Read the model definition and answer for the solid it produces. Units are mm, in the model's axes. A direction names the side the tool comes from. Give positions to 0.01 mm unless a question says otherwise; leave off trailing zeros. Order: outer loops, then holes, each group sorted by start corner. A loop starts at its lowest first (then second) coordinate and runs counter-clockwise, first axis right, second up. Notation, with made-up numbers: M 39,-1.75 L 70,-1.75 A34 ccw 70,29.25 Z; hole C 19,83.5 d5. An arc over 180 degrees is marked long. Write item = value, one per line. Start each with the question number.
from build123d import *

# Parameters (mm, degrees)
SKETCH2_W           = 120
SKETCH2_H           = 105
SKETCH2_R           = 1.4
BOSS_EXTRUDE2_DEPTH = 5
CUT_EXTRUDE13_DEPTH = 90.336442732
FILLET6_R           = 5
FILLET5_R           = 10
CHAMFER4_SIZE       = 1
SKETCH11_R          = 2.15
CUT_EXTRUDE10_DEPTH = 90.336442732
SKETCH13_R          = 3.25
CUT_EXTRUDE12_DEPTH = 2.5
CUT_EXTRUDE14_DEPTH = 90.336442732
CHAMFER5_SIZE       = 3
CHAMFER5_SIZE_2     = 8.242432258


with BuildPart() as part:
    # Sketch2 → Boss-Extrude2 (new body)
    with BuildSketch(Plane(origin=(0, 0, 0), x_dir=(1, 0, 0), z_dir=(0, 1, 0))):
        with Locations((0, 13.5)):
            Rectangle(SKETCH2_W, SKETCH2_H)
        with Locations(Location((-28, -28, 0), (0, 0, 270))):
            Circle(SKETCH2_R, mode=Mode.SUBTRACT)
        with Locations(Location((28, -28, 0), (0, 0, 270))):
            Circle(SKETCH2_R, mode=Mode.SUBTRACT)
        with Locations(Location((20, 42, 0), (0, 0, 270))):
            Circle(SKETCH2_R, mode=Mode.SUBTRACT)
        with Locations(Location((-20, 42, 0), (0, 0, 270))):
            Circle(SKETCH2_R, mode=Mode.SUBTRACT)
    extrude(amount=BOSS_EXTRUDE2_DEPTH)

    # Sketch9 → Cut-Extrude13 (cut, through all)
    with BuildSketch(Plane(origin=(0, 5, 0), x_dir=(1, 0, 0), z_dir=(0, 1, 0))):
        Polygon((-26, 66), (-20, 60), (20, 60), (26, 66), align=None)
    extrude(amount=-CUT_EXTRUDE13_DEPTH, mode=Mode.SUBTRACT)

    # Fillet6
    fillet6_edges = [part.edges().sort_by_distance(p)[0] for p in [
        (-26, 2.5, -66),
        (26, 2.5, -66),
        (20, 2.5, -60),
        (-20, 2.5, -60),
    ]]
    fillet(fillet6_edges, radius=FILLET6_R)

    # Fillet5
    fillet5_edges = [part.edges().sort_by_distance(p)[0] for p in [
        (-60, 2.5, -66),
        (60, 2.5, -66),
        (60, 2.5, 39),
        (-60, 2.5, 39),
    ]]
    fillet(fillet5_edges, radius=FILLET5_R)

    # Chamfer4
    chamfer4_edges = [part.edges().sort_by_distance(p)[0] for p in [
        (23, 5, -63),
        (0, 5, -60),
        (-23, 5, -63),
        (-39.035533906, 5, -66),
        (-26.15765065, 5, -65.619397663),
        (26.15765065, 5, -65.619397663),
        (19.84234935, 5, -60.380602337),
        (-19.84234935, 5, -60.380602337),
        (-60, 5, -13.5),
        (39.035533906, 5, -66),
        (0, 5, 39),
        (60, 5, -13.5),
        (-57.071067812, 5, 36.071067812),
        (57.071067812, 5, 36.071067812),
        (57.071067812, 5, -63.071067812),
        (-57.071067812, 5, -63.071067812),
    ]]
    chamfer(chamfer4_edges, length=CHAMFER4_SIZE)

    # Sketch11 → Cut-Extrude10 (cut, through all)
    with BuildSketch(Plane(origin=(0, 5, 0), x_dir=(1, 0, 0), z_dir=(0, 1, 0))):
        with Locations(Location((-50, 56, 0), (0, 0, 270))):
            Circle(SKETCH11_R)
        with Locations(Location((50, 56, 0), (0, 0, 270))):
            Circle(SKETCH11_R)
        with Locations(Location((-50, -19, 0), (0, 0, 270))):
            Circle(SKETCH11_R)
        with Locations(Location((50, -19, 0), (0, 0, 270))):
            Circle(SKETCH11_R)
    extrude(amount=-CUT_EXTRUDE10_DEPTH, mode=Mode.SUBTRACT)

    # Sketch13 → Cut-Extrude12 (cut)
    with BuildSketch(Plane.XZ):
        with Locations(Location((-28, 28, 0), (0, 0, 270))):
            Circle(SKETCH13_R)
        with Locations(Location((28, 28, 0), (0, 0, 270))):
            Circle(SKETCH13_R)
        with Locations(Location((-20, -42, 0), (0, 0, 270))):
            Circle(SKETCH13_R)
        with Locations(Location((20, -42, 0), (0, 0, 270))):
            Circle(SKETCH13_R)
    extrude(amount=-CUT_EXTRUDE12_DEPTH, mode=Mode.SUBTRACT)

    # Sketch14 → Cut-Extrude14 (cut, through all)
    with BuildSketch(Plane(origin=(0, 5, 0), x_dir=(1, 0, 0), z_dir=(0, 1, 0))):
        with BuildLine():
            Line((-11, 38), (11, 38))
            ThreePointArc((11, 38), (18, 31), (11, 24))
            Line((11, 24), (-11, 24))
            ThreePointArc((-11, 24), (-18, 31), (-11, 38))
        make_face()
    extrude(amount=-CUT_EXTRUDE14_DEPTH, mode=Mode.SUBTRACT)

    # Chamfer5
    # the kernel refuses this chamfer: 8.242432258, 3 mm, written as the material it takes off along each edge
    with BuildSketch(Plane(origin=(11, 5, -24), x_dir=(0, 0.09904090225205062, 0.9950833631817486), z_dir=(-1, 0, 0)), Plane(origin=(-11, 5, -38), x_dir=(0, 0.09904090225205073, -0.9950833631817486), z_dir=(1, 0, 0))) as chamfer5_piece_1:
        Polygon((CHAMFER5_SIZE * 0.995083363182, -CHAMFER5_SIZE * 0.0990409022521), (-CHAMFER5_SIZE_2 * 0.0990409022564, -CHAMFER5_SIZE_2 * 0.995083363226), (0, 0), align=None)
    extrude(amount=22, mode=Mode.SUBTRACT)
    with BuildSketch(Plane(origin=(11, 5, -31), x_dir=(0, 0, -1), z_dir=(-1, 0, 0))) as chamfer5_piece_2:
        Polygon((7 + CHAMFER5_SIZE, 0), (7, CHAMFER5_SIZE_2), (7, 0), align=None)
    revolve(axis=Axis((11, 5, -31), (0, -1, 0)), revolution_arc=180, mode=Mode.SUBTRACT)
    with BuildSketch(Plane(origin=(-11, 5, -31), x_dir=(0, 0, 1), z_dir=(1, 0, 0))) as chamfer5_piece_3:
        Polygon((7 + CHAMFER5_SIZE, 0), (7, CHAMFER5_SIZE_2), (7, 0), align=None)
    revolve(axis=Axis((-11, 5, -31), (0, -1, 0)), revolution_arc=180, mode=Mode.SUBTRACT)


solid = part.part
1) Find section A-A on z = -31. Determine the outline of the cut face in (x, y).
2) Find section B-B on x = 9. Determine the outline of the cut face in (y, z), plus the area to 3 significant figures.
3) For a pull along X with two mould halves and no side action, classify faces 6 (the face through (-56.558, 4.826, -62.415)), 7 (the face through (26.6, 2.5, 27.3)), 8 (the face through (39, 2, -66)) as pulls with the +X half, pulls with the -X half, needs draft (parallel to the pull), parting line crosses it, or undercut.
4) For faces 1 (the face through (-19.87, 1.97, -60.39)), 2 (the face through (19.67, 1.35, -31.19)), 3 (the face through (-20.02, 4.38, -60.04)), 4 (the face through (25.117, 1.232, 26.5)), 5 (the face through (-27.94, 3.73, 26.6)), determine the directions among +Z, -Z, +X, -X, +Y, -Y from which every point of the face is accessible in a straight line to the end or side of a thin tool.
5) Find the intervals of material crossed by probe 1 along X at (y, z) = (1.65, -56); probe 2 along X at (y, z) = (1.75, -42); probe 3 along Z at (x, y) = (-50.5, 0.75), in increasing order. Write a range as [from, to].
6) Each of these flat-tipped pins is pushed along its axis until it touches: P1, Ø3, axis at x = 6.5, y = 2, coming from the -Z side; P2, Ø3, axis at x = -28, z = 28, coming from the -Y side; P3, Ø1.7, axis at x = -20, z = -42, coming from the -Y side. Where does it stop, or does it pass through?
Numbers:
q1.outline = M -60,0 L -19.18,0 L -21,5 L -59,5 L -60,4 Z; M 19.18,0 L 60,0 L 60,4 L 59,5 L 21,5 Z
q2.outline = M 0,-60 L 4,-60 L 5,-59 L 5,-41 L 0,-39.18 Z; M 0,-22.82 L 5,-21 L 5,38 L 4,39 L 0,39 Z
q2.area = 403 mm2
q3.face_6 = pulls with the -X half
q3.face_7 = undercut
q3.face_8 = needs draft
q4.face_1 = -Z, +Y, -Y
q4.face_2 = +Y
q4.face_3 = -Z, +Y
q4.face_4 = -Y
q4.face_5 = +Y, -Y
q5.probe_1 = [-60, -52.15], [-47.85, 47.85], [52.15, 60]
q5.probe_2 = [-60, -23.25], [-16.75, 16.75], [23.25, 60]
q5.probe_3 = [-65.99, -58.09], [-53.91, 16.91], [21.09, 38.99]
q6.P1 = -60
q6.P2 = 2.5
q6.P3 = through
